CAD build for the part. Positions are in the model's coordinates, mm. Face numbers are marked on the shaded views. A direction names the side the tool comes from. Coordinates: 2 decimals unless noted, no trailing zeros. Order: outer loops, then holes, each group sorted by start corner. A loop starts at its lowest first (then second) coordinate and runs counter-clockwise, first axis right, second up. Notation, with made-up numbers: (-25, 6.25) - (-8, 6.25) arc R24 ccw to (-8, 42.25) - close; hole circle Ø8 at (-6, 31.5). An arc over 180 degrees is marked (long way). Return JSON: item names as keys, results as strings.
from build123d import *

# Parameters (mm, degrees)
F0_R         = 9.525
F0_W         = 38.1
F0_H         = 14.8362964392
F1_DEPTH     = 25.4
F2_R         = 5.08
F3_T1_DEPTH  = 15.24
F3_S5_W      = 5.08
F3_S5_H      = 5.08
F3_T6_DEPTH  = 5.08
F3_S11_W     = 5.08
F3_S11_H     = 5.08
F3_T12_DEPTH = 5.08
F3_S17_W     = 5.08
F3_S17_H     = 5.08
F3_T18_DEPTH = 5.08
F3_S23_W     = 5.08
F3_S23_H     = 5.08
F3_T24_DEPTH = 5.08


# Not quite as in the source:
# - a fillet or chamfer that OpenCascade refuses, or shapes differently, is made with other operations: its cross-section is extruded or revolved along the edge and cut away or added


with BuildPart() as f1:
    # F0 (on Top) → F1 (new body)
    with BuildSketch(Plane.XY):
        Polygon((-105.0124109644, 7.0207449608), (-66.9124109644, 7.0207449608), (-66.9124109644, 19.73756589), (-66.9124109644, 34.5738623291), (-66.9124109644, 45.1207449608), (-105.0124109644, 45.1207449608), align=None)
        with Locations((-85.9624109644, 26.0707449608)):
            Circle(F0_R, mode=Mode.SUBTRACT)
        with Locations((-47.8624109644, 27.1557141095)):
            Rectangle(F0_W, F0_H)
        Polygon((-28.8124109644, 34.5738623291), (-28.8124109644, 19.73756589), (-28.8124109644, 7.0207449608), (9.2875890356, 7.0207449608), (9.2875890356, 45.1207449608), (-28.8124109644, 45.1207449608), align=None)
        with Locations((-9.7624109644, 26.0707449608)):
            Circle(F0_R, mode=Mode.SUBTRACT)
    extrude(amount=F1_DEPTH)

    # F2
    f2_edges = [f1.edges().sort_by_distance(p)[0] for p in [
        (-85.962411, 45.120745, 25.4),
        (-85.962411, 45.120745, 0),
        (-105.012411, 45.120745, 12.7),
        (-105.012411, 26.070745, 0),
        (-105.012411, 26.070745, 25.4),
        (-85.962411, 7.020745, 25.4),
        (-47.862411, 19.737566, 25.4),
        (-47.862411, 34.573862, 25.4),
        (-66.912411, 39.847304, 25.4),
        (-66.912411, 13.379155, 25.4),
        (-28.812411, 13.379155, 25.4),
        (-9.762411, 7.020745, 25.4),
        (9.287589, 26.070745, 25.4),
        (-9.762411, 45.120745, 25.4),
        (9.287589, 7.020745, 12.7),
        (9.287589, 45.120745, 12.7),
        (9.287589, 26.070745, 0),
        (-47.862411, 19.737566, 0),
        (-66.912411, 13.379155, 0),
        (-66.912411, 7.020745, 12.7),
        (-28.812411, 7.020745, 12.7),
        (-85.962411, 7.020745, 0),
        (-47.862411, 34.573862, 0),
        (-9.762411, 45.120745, 0),
        (-28.812411, 45.120745, 12.7),
        (-28.812411, 39.847304, 0),
        (-66.912411, 39.847304, 0),
        (-9.762411, 7.020745, 0),
        (-28.812411, 13.379155, 0),
    ]]
    fillet(f2_edges, radius=F2_R)

    # F3: fillet of radius 5.08 on 2 edges, made by hand

    # F3_s2 → F3_t1 (cut)
    with BuildSketch(Plane.XY.offset(5.08)):
        with BuildLine():
            ThreePointArc((-71.9924109644, 45.1207449608), (-68.4003085159, 43.6328474092), (-66.9124109644, 40.0407449608))
            Line((-66.9124109644, 40.0407449608), (-66.9124109644, 45.1207449608))
            Line((-66.9124109644, 45.1207449608), (-71.9924109644, 45.1207449608))
        make_face()
        with BuildLine():
            ThreePointArc((-105.0124109644, 12.1007449608), (-103.5245134128, 8.5086425123), (-99.9324109644, 7.0207449608))
            Line((-99.9324109644, 7.0207449608), (-105.0124109644, 7.0207449608))
            Line((-105.0124109644, 7.0207449608), (-105.0124109644, 12.1007449608))
        make_face()
    extrude(amount=F3_T1_DEPTH, mode=Mode.SUBTRACT)


with BuildPart() as f3_tool4:
    # F3_s5 → F3_t6 (new body)
    with BuildSketch(Plane.YZ.offset(-99.9324109644)):
        with Locations((9.5607449608, 2.54)):
            Rectangle(F3_S5_W, F3_S5_H)
    extrude(amount=-F3_T6_DEPTH)

    # F3_s7 → F3_t8 (revolve, cut)
    with BuildSketch(Plane(origin=(-99.9324109644, 12.1007449608, 5.08), x_dir=(0, 0.7071067812, 0.7071067812), z_dir=(0, -0.7071067812, 0.7071067812))):
        with BuildLine():
            ThreePointArc((0, -5.08), (5.08, 0), (0, 5.08))
            Line((0, 5.08), (0, -5.08))
        make_face()
    revolve(axis=Axis((-99.9324109644, 12.1007449608, 5.08), (-1, 0, 0)), mode=Mode.SUBTRACT)


with BuildPart() as f1_1:
    add(f1.part)

    # F3_t3: cut F3_tool4
    add(f3_tool4.part, mode=Mode.SUBTRACT)


with BuildPart() as f3_tool10:
    # F3_s11 → F3_t12 (new body)
    with BuildSketch(Plane.YZ.offset(-99.9324109644)):
        with Locations((9.5607449608, 22.86)):
            Rectangle(F3_S11_W, F3_S11_H)
    extrude(amount=-F3_T12_DEPTH)

    # F3_s13 → F3_t14 (revolve, cut)
    with BuildSketch(Plane(origin=(-99.9324109644, 12.1007449608, 20.32), x_dir=(0, 0.7071067812, -0.7071067812), z_dir=(0, 0.7071067812, 0.7071067812))):
        with BuildLine():
            ThreePointArc((0, -5.08), (5.08, 0), (0, 5.08))
            Line((0, 5.08), (0, -5.08))
        make_face()
    revolve(axis=Axis((-99.9324109644, 12.1007449608, 20.32), (-1, 0, 0)), mode=Mode.SUBTRACT)


with BuildPart() as f1_2:
    add(f1_1.part)

    # F3_t9: cut F3_tool10
    add(f3_tool10.part, mode=Mode.SUBTRACT)


with BuildPart() as f3_tool16:
    # F3_s17 → F3_t18 (new body)
    with BuildSketch(Plane.XZ.offset(-40.0407449608)):
        with Locations((-69.4524109644, 2.54)):
            Rectangle(F3_S17_W, F3_S17_H)
    extrude(amount=-F3_T18_DEPTH)

    # F3_s19 → F3_t20 (revolve, cut)
    with BuildSketch(Plane(origin=(-71.9924109644, 40.0407449608, 5.08), x_dir=(-0.7071067812, 0, 0.7071067812), z_dir=(-0.7071067812, 0, -0.7071067812))):
        with BuildLine():
            ThreePointArc((0, -5.08), (5.08, 0), (0, 5.08))
            Line((0, 5.08), (0, -5.08))
        make_face()
    revolve(axis=Axis((-71.9924109644, 40.0407449608, 5.08), (0, 1, 0)), mode=Mode.SUBTRACT)


with BuildPart() as f1_3:
    add(f1_2.part)

    # F3_t15: cut F3_tool16
    add(f3_tool16.part, mode=Mode.SUBTRACT)


with BuildPart() as f3_tool22:
    # F3_s23 → F3_t24 (new body)
    with BuildSketch(Plane.XZ.offset(-40.0407449608)):
        with Locations((-69.4524109644, 22.86)):
            Rectangle(F3_S23_W, F3_S23_H)
    extrude(amount=-F3_T24_DEPTH)

    # F3_s25 → F3_t26 (revolve, cut)
    with BuildSketch(Plane(origin=(-71.9924109644, 40.0407449608, 20.32), x_dir=(-0.7071067812, 0, -0.7071067812), z_dir=(0.7071067812, 0, -0.7071067812))):
        with BuildLine():
            ThreePointArc((0, -5.08), (5.08, 0), (0, 5.08))
            Line((0, 5.08), (0, -5.08))
        make_face()
    revolve(axis=Axis((-71.9924109644, 40.0407449608, 20.32), (0, 1, 0)), mode=Mode.SUBTRACT)


with BuildPart() as f1_4:
    add(f1_3.part)

    # F3_t21: cut F3_tool22
    add(f3_tool22.part, mode=Mode.SUBTRACT)


solid = f1_4.part
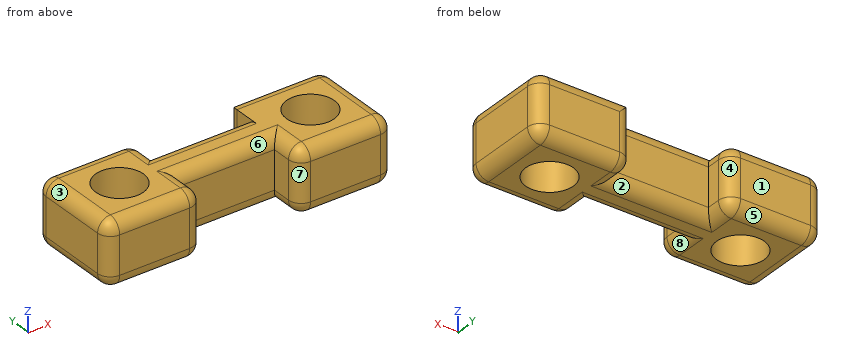
Item 1: Mould opens along X. For the marked faces 1, 2 and 3 say: released by +X, released by -X, zero draft, split by the parting line, or undercut.
Findings below:
{"face 1": "zero draft", "face 2": "undercut", "face 3": "released by -X"}
Item 2: Band-saw the part on D-D, the plane z = 23. List the corners of the cut face in (x, y) (3 decimals).
Findings below:
{"outline": "(-104.248, 12.101) arc R4.316 ccw to (-99.932, 7.785) - (-71.992, 7.785) arc R4.316 ccw to (-67.677, 12.101) - (-67.677, 20.502) - (-28.048, 20.502) - (-28.048, 12.101) arc R4.316 ccw to (-23.732, 7.785) - (4.208, 7.785) arc R4.316 ccw to (8.523, 12.101) - (8.523, 40.041) arc R4.316 ccw to (4.208, 44.356) - (-26.412, 44.356) arc R5.08 ccw to (-28.812, 40.041) - (-28.812, 33.809) - (-67.677, 33.809) - (-67.677, 40.041) arc R4.316 ccw to (-71.992, 44.356) - (-99.932, 44.356) arc R4.316 ccw to (-104.248, 40.041) - close; hole circle Ø19.05 at (-85.962, 26.071); hole circle Ø19.05 at (-9.762, 26.071)"}
Item 3: Band-saw the part on B-B, the plane y = 10.5. List the corners of the cut face in (x, z).
Findings below:
{"outline": "(-104.75, 5.08) arc R4.82 ccw to (-99.93, 0.26) - (-71.99, 0.26) arc R4.82 ccw to (-67.17, 5.08) - (-67.17, 20.32) arc R4.82 ccw to (-71.99, 25.14) - (-99.93, 25.14) arc R4.82 ccw to (-104.75, 20.32) - close; (-28.55, 5.08) arc R4.82 ccw to (-23.73, 0.26) - (4.21, 0.26) arc R4.82 ccw to (9.03, 5.08) - (9.03, 20.32) arc R4.82 ccw to (4.21, 25.14) - (-23.73, 25.14) arc R4.82 ccw to (-28.55, 20.32) - close"}
Item 4: Drop flat-ended pins along their axis: P1, Ø12, axis at x = -14, y = 27.5, coming from the -Z side; P2, Ø7.5, axis at x = -52, z = 9.5, coming from the -Y side; P3, Ø12, axis at x = -42.5, z = 13, coming from the +Y side; P4, Ø3, axis at x = -66.5, y = 33.5, coming from the -Z side. Give the stop position or say it passes through.
Findings below:
{"P1": "stops at z = 0", "P2": "stops at y = 19.74", "P3": "stops at y = 34.57", "P4": "stops at z = 0.66"}
Item 5: Band-saw the part on A-A, the plane x = -64.5. List the corners of the cut face in (y, z), then the cut area to 3 significant figures.
Findings below:
{"outline": "(19.74, 5.08) arc R5.08 ccw to (24.82, 0) - (29.49, 0) arc R5.08 ccw to (34.57, 5.08) - (34.57, 20.32) arc R5.08 ccw to (29.49, 25.4) - (24.82, 25.4) arc R5.08 ccw to (19.74, 20.32) - close", "area": "355 mm²"}
Item 6: Which spindle directions (+Z, -Z, +X, -X, +Y, -Y) get a long thin tool onto all of the face, cutting with end or side? Do the marked faces 4, 5, 6, 7 and 8. Say none if no direction does.
Findings below:
{"face 4": "+Z, -Z, +Y", "face 5": "-Z, +X, -X, +Y", "face 6": "+Z, -Y", "face 7": "+Z, -Z, -Y", "face 8": "-Z, -Y"}
Item 7: Wall check: L1, parallel to X at y = 26, z = 18.5; L2, parallel to X at y = 12, z = 7; L3, parallel to X at y = 31.5, z = 9. Give the ranges that are in metal, low to high. Write a range as [from, to].
Findings below:
{"L1": "x = [-105.01, -95.49], [-76.44, -19.29], [-0.24, 9.29]", "L2": "x = [-105.01, -66.91], [-28.81, 9.29]", "L3": "x = [-105.01, -93.79], [-78.14, -17.59], [-1.94, 9.29]"}
Item 8: Band-saw the part on C-C, the plane x = -84.5. List the corners of the cut face in (y, z), then the cut area to 3 significant figures.
Findings below:
{"outline": "(7.02, 5.08) arc R5.08 ccw to (12.1, 0) - (16.66, 0) - (16.66, 25.4) - (12.1, 25.4) arc R5.08 ccw to (7.02, 20.32) - close; (35.48, 0) - (40.04, 0) arc R5.08 ccw to (45.12, 5.08) - (45.12, 20.32) arc R5.08 ccw to (40.04, 25.4) - (35.48, 25.4) - close", "area": "467 mm²"}
